from build123d import *

# Parameters (mm, degrees)
F0_W     = 152
F0_H     = 50
F1_DEPTH = 2


with BuildPart() as f1:
    # F0 (on Front) → F1 (new body)
    with BuildSketch(Plane.XZ):
        with Locations((76, 25)):
            Rectangle(F0_W, F0_H)
        Polygon((29.780989, 6), (6, 6), (6, 37.377694), (6, 44), (30.8, 44), (34.8, 44), (59.6, 44), (63.6, 44), (88.4, 44), (92.4, 44), (117.2, 44), (121.2, 44), (146, 44), (150, 44), (150, 6), (144.980989, 6), (121.2, 6), (116.180989, 6), (92.4, 6), (87.380989, 6), (63.6, 6), (58.580989, 6), (34.8, 6), align=None, mode=Mode.SUBTRACT)
        Polygon((121.2, 37.377694), (144.980989, 6), (150, 6), (146, 11.277778), (121.2, 44), align=None)
        Polygon((117.2, 11.277778), (121.2, 6), (121.2, 37.377694), (121.2, 44), (117.2, 44), align=None)
        Polygon((92.4, 37.377694), (116.180989, 6), (121.2, 6), (117.2, 11.277778), (92.4, 44), align=None)
        Polygon((88.4, 11.277778), (92.4, 6), (92.4, 37.377694), (92.4, 44), (88.4, 44), align=None)
        Polygon((63.6, 37.377694), (87.380989, 6), (92.4, 6), (88.4, 11.277778), (63.6, 44), align=None)
        Polygon((59.6, 11.277778), (63.6, 6), (63.6, 37.377694), (63.6, 44), (59.6, 44), align=None)
        Polygon((34.8, 37.377694), (58.580989, 6), (63.6, 6), (59.6, 11.277778), (34.8, 44), align=None)
        Polygon((30.8, 11.277778), (34.8, 6), (34.8, 37.377694), (34.8, 44), (30.8, 44), align=None)
        Polygon((6, 37.377694), (29.780989, 6), (34.8, 6), (30.8, 11.277778), (6, 44), align=None)
        Polygon((146, 11.277778), (150, 6), (150, 44), (146, 44), align=None)
    extrude(amount=F1_DEPTH)


solid = f1.part
CAD build for the part. Positions are in the model's coordinates, mm. A direction names the side the tool comes from. Round coordinates to 2 decimals unless told otherwise and drop trailing zeros. Order: outer loops, then holes, each group sorted by start corner. A loop starts at its lowest first (then second) coordinate and runs counter-clockwise, first axis right, second up. Notation, with made-up numbers: (-1.5, -11) - (41.5, -11) arc R30 ccw to (41.5, 17) - close; hole circle Ø2 at (52, 84.5). An arc over 180 degrees is marked (long way). Return JSON: item names as keys, results as strings.
(1) Cut at B-B (x = 97). Give the cut face in (y, z), then the cut area to 3 significant figures.
Answer key:
{"outline": "(-2, 0) - (0, 0) - (0, 6) - (-2, 6) - close; (-2, 31.31) - (0, 31.31) - (0, 37.93) - (-2, 37.93) - close; (-2, 44) - (0, 44) - (0, 50) - (-2, 50) - close", "area": "37.2 mm^2"}
(2) Tool access for faces 1 (the face through (75, 0, 25)), 2 (the face through (104.974, -0.986, 27.41)): list every direction of +Z, -Z, +X, -X, +Y, -Y with a clear straight run to the whole face (end or side of a thin tool).
Answer key:
{"face 1": "+Z, -Z, +X, -X, +Y", "face 2": "+Y, -Y"}
(3) Pull direction X, two halves, no side cores. Call faces 3 (the face through (75, -2, 25)), 4 (the face through (75.324, -0.986, 21.908)): +X half, -X half, draft (parallel to the pull), parting line (faces both ways), or undercut.
Answer key:
{"face 3": "draft", "face 4": "undercut"}
(4) Cut at C-C (z = 40.5). Give the cut face in (x, y), then the cut area to 3 significant figures.
Answer key:
{"outline": "(0, -2) - (8.65, -2) - (8.65, 0) - (0, 0) - close; (30.8, -2) - (37.45, -2) - (37.45, 0) - (30.8, 0) - close; (59.6, -2) - (66.25, -2) - (66.25, 0) - (59.6, 0) - close; (88.4, -2) - (95.05, -2) - (95.05, 0) - (88.4, 0) - close; (117.2, -2) - (123.85, -2) - (123.85, 0) - (117.2, 0) - close; (146, -2) - (152, -2) - (152, 0) - (146, 0) - close", "area": "82.5 mm^2"}
(5) Wall check: probe 1 along Z at (x, y) = (143, -0.9); probe 2 along Z at (x, y) = (109.5, -1.85). Give the ranges that are in metal, low to high. Write a range as from..to.
Answer key:
{"probe 1": "z = 0..6, 8.61..15.24, 44..50", "probe 2": "z = 0..6, 14.82..21.44, 44..50"}
(6) Cut at A-A (y = -1.3). State how many separate pieces and enclosed holes the cut face has, then the cut area to 3 significant figures.
Answer key:
{"separate pieces": "1", "enclosed holes": "10", "area": "3,710 mm^2"}
